```python
from build123d import *

# Parameters (mm, degrees)
SKETCH1_R           = 3.175
BOSS_EXTRUDE1_DEPTH = 2.54


with BuildPart() as part:
    # Sketch1 → Boss-Extrude1 (new body)
    # profile 1 of 5: a face of its own
    with BuildSketch(Plane(origin=(0, 0, 0), x_dir=(1, 0, 0), z_dir=(0, 1, 0))):
        with BuildLine():
            ThreePointArc((-7.099515829, -6.35), (-9.525, 0), (-7.099515829, 6.35))
            Line((-7.099515829, 6.35), (-38.1, 6.35))
            Line((-38.1, 6.35), (-38.1, -6.35))
            Line((-38.1, -6.35), (-7.099515829, -6.35))
        make_face()
        with Locations(Location((-31.75, 0, 0), (0, 0, 270))):
            Circle(SKETCH1_R, mode=Mode.SUBTRACT)
    # profile 2 of 5: a face of its own
    with BuildSketch(Plane(origin=(0, 0, 0), x_dir=(1, 0, 0), z_dir=(0, 1, 0))):
        with BuildLine():
            Line((0, -6.35), (0, 0))
            Line((0, 0), (0, 6.35))
            Line((0, 6.35), (-7.099515829, 6.35))
            ThreePointArc((-7.099515829, 6.35), (-9.525, 0), (-7.099515829, -6.35))
            Line((-7.099515829, -6.35), (0, -6.35))
        make_face()
    # profile 3 of 5: a face of its own
    with BuildSketch(Plane(origin=(0, 0, 0), x_dir=(1, 0, 0), z_dir=(0, 1, 0))):
        with BuildLine():
            Line((0, 6.35), (0, 0))
            Line((0, 0), (0, -6.35))
            Line((0, -6.35), (-7.099515829, -6.35))
            ThreePointArc((-7.099515829, -6.35), (3.398730405, -8.897991719), (9.525, 0))
            ThreePointArc((9.525, 0), (3.398730405, 8.897991719), (-7.099515829, 6.35))
            Line((-7.099515829, 6.35), (0, 6.35))
        make_face()
    # profile 4 of 5: a face of its own
    with BuildSketch(Plane(origin=(0, 0, 0), x_dir=(1, 0, 0), z_dir=(0, 1, 0))):
        with BuildLine():
            Line((0, -6.35), (0, 0))
            Line((0, 0), (0, 6.35))
            Line((0, 6.35), (-7.099515829, 6.35))
            ThreePointArc((-7.099515829, 6.35), (-9.525, 0), (-7.099515829, -6.35))
            Line((-7.099515829, -6.35), (0, -6.35))
        make_face()
    # profile 5 of 5: a face of its own
    with BuildSketch(Plane(origin=(0, 0, 0), x_dir=(1, 0, 0), z_dir=(0, 1, 0))):
        with BuildLine():
            Line((0, 6.35), (0, 0))
            Line((0, 0), (0, -6.35))
            Line((0, -6.35), (-7.099515829, -6.35))
            ThreePointArc((-7.099515829, -6.35), (3.398730405, -8.897991719), (9.525, 0))
            ThreePointArc((9.525, 0), (3.398730405, 8.897991719), (-7.099515829, 6.35))
            Line((-7.099515829, 6.35), (0, 6.35))
        make_face()
    extrude(amount=BOSS_EXTRUDE1_DEPTH)


solid = part.part
```
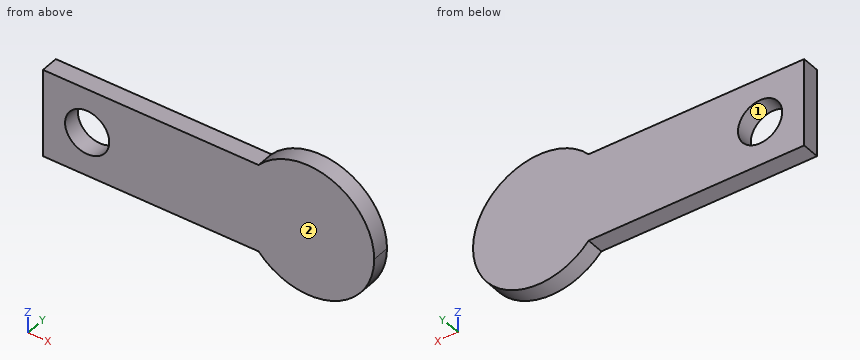
The listing builds one solid part. Answer for the finished solid, in the listing's coordinates (mm). Face numbers are marked on the shaded views. Give positions to 0.01 mm unless a question says otherwise; leave off trailing zeros. Order: outer loops, then holes, each group sorted by start corner. A loop starts at its lowest first (then second) coordinate and runs counter-clockwise, first axis right, second up.
1) Find section B-B on z = -1.75. Write down the section's boundary in (x, y).
Reported:
outline: (-38.1, 0) - (-34.4, 0) - (-34.4, 2.54) - (-38.1, 2.54) - close; (-29.1, 0) - (9.36, 0) - (9.36, 2.54) - (-29.1, 2.54) - close
2) Consider line 1 along Z through (x, y) = (-7.5, 2.2); line 2 along Z through (x, y) = (-31, 0.55); line 3 along X through (y, z) = (1.4, -1). Determine where each line is inside the solid, lowest interval first.
Reported:
line 1: z = -6.35 to 6.35
line 2: z = -6.35 to -3.09, 3.09 to 6.35
line 3: x = -38.1 to -34.76, -28.74 to 9.47
3) Find section A-A on x = -31.75. Write down the section's boundary in (y, z) (3 decimals), then the cut area to 3 significant figures.
Reported:
outline: (0, -6.35) - (2.54, -6.35) - (2.54, -3.175) - (0, -3.175) - close; (0, 3.175) - (2.54, 3.175) - (2.54, 6.35) - (0, 6.35) - close
area: 16.1 mm2
4) Given P1, Ø1.5, axis at x = -24, z = 7.5, coming from the -Y side; P2, Ø0.8, axis at x = -28, y = 1.5, coming from the -Z side; P3, Ø1.3, axis at x = -23, y = 1, coming from the +Z side, each flat-ended and moving along its own axis, determine where each tip first touches the part or whether it passes through.
Reported:
P1: passes through
P2: stops at z = -6.35
P3: stops at z = 6.35
5) Determine the mould class of the marked faces 1 and 2 for opening direction Z: pulls with the +Z half, pulls with the -Z half, needs draft (parallel to the pull), parting line crosses it, or undercut.
Reported:
face 1: undercut
face 2: needs draft
6) Find section C-C on y = 0.95. Write down the section's boundary in (x, z) (3 decimals).
Reported:
outline: (-38.1, -6.35) - (-7.1, -6.35) arc R9.525 ccw (long way) to (-7.1, 6.35) - (-38.1, 6.35) - close; hole circle Ø6.35 at (-31.75, 0)
7) Find section D-D on x = -15.5. Write down the section's boundary in (y, z), then the cut area to 3 significant figures.
Reported:
outline: (0, -6.35) - (2.54, -6.35) - (2.54, 6.35) - (0, 6.35) - close
area: 32.3 mm2
